Read the model definition and answer for the solid it produces. Units are mm, in the model's axes. Face numbers are marked on the shaded views. A direction names the side the tool comes from. Round coordinates to 2 decimals unless told otherwise and drop trailing zeros. Order: outer loops, then holes, each group sorted by start corner. A loop starts at its lowest first (then second) coordinate and runs counter-clockwise, first axis right, second up.
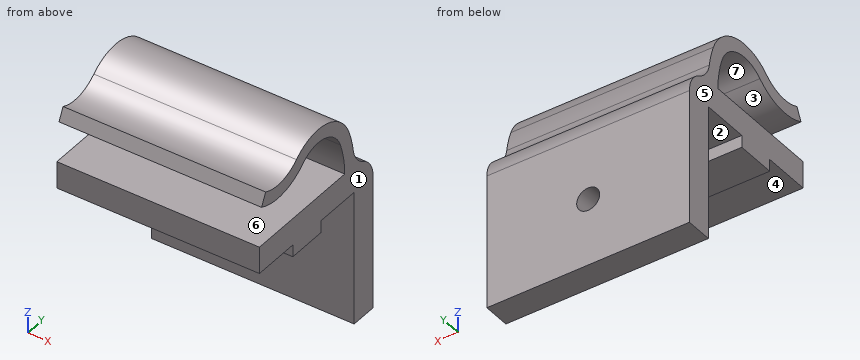
from build123d import *

# Parameters (mm, degrees)
PAD018_DEPTH    = 15
FILLET017_R     = 4
SKETCH077_R     = 1.7
POCKET041_DEPTH = 14.0010001


with BuildPart() as part:
    # Sketch076 → Pad018 (new body, symmetric)
    with BuildSketch(Plane.YZ):
        with BuildLine():
            Line((-2.95, 0), (2.95, 0))
            Line((2.95, 0), (2.95, 1.8))
            Line((2.95, 1.8), (10, 1.8))
            Line((10, -18.2), (10, 1.8))
            Line((14, -18.2), (10, -18.2))
            Line((14, 1.8), (14, -18.2))
            ThreePointArc((14, 1.8), (12.8284271247, 4.6284271247), (10, 5.8))
            ThreePointArc((10, 5.8), (9.7359108307, 8.6950147374), (8.9523612088, 11.4944617201))
            ThreePointArc((8.9523612088, 11.4944617201), (4.1074030924, 15.7943944981), (-2.1905894743, 14.2783698696))
            ThreePointArc((-8.6955362552, 13.3740094918), (-5.3083417089, 12.8571578981), (-2.1905894743, 14.2783698696))
            Line((-9.5491968047, 11.565345989), (-8.6955362552, 13.3740094918))
            ThreePointArc((-9.5491968047, 11.565345989), (-5.0329374097, 10.8762105308), (-0.8759344302, 12.7711598262))
            ThreePointArc((7.0833160577, 10.7826540051), (3.6226316889, 13.8540345608), (-0.8759344302, 12.7711598262))
            ThreePointArc((8, 5.8), (7.7689219768, 8.3331378952), (7.0833160577, 10.7826540051))
            Line((-10, 5.8), (8, 5.8))
            Line((-10, 5.8), (-10, 1.8))
            Line((-2.95, 1.8), (-10, 1.8))
            Line((-2.95, 0), (-2.95, 1.8))
        make_face()
    extrude(amount=PAD018_DEPTH, both=True)

    # Fillet017
    fillet017_edges = [part.edges().sort_by_distance(p)[0] for p in [
        (0, 10, 5.8),
    ]]
    fillet(fillet017_edges, radius=FILLET017_R)

    # Sketch077 → Pocket041 (cut, through all)
    with BuildSketch(Plane.XZ):
        with Locations((0, -8.2)):
            Circle(SKETCH077_R)
    extrude(amount=-POCKET041_DEPTH, mode=Mode.SUBTRACT)


solid = part.part
Q1. For a pull along Z with two mould halves and no side action, classify the marked faces 1, 2 and 3 as released by +Z, released by -Z, zero draft, split by the parting line, or undercut.
Outcome:
face 1: zero draft
face 2: released by -Z
face 3: undercut
Q2. For the marked faces 4, 5, 6 and 7, determine the directions among +Z, -Z, +X, -X, +Y, -Y from which every point of the face is accessible in a straight line to the end or side of a thin tool.
Outcome:
face 4: -Z, +X, -X, -Y
face 5: +Z, -Z, -X, +Y, -Y
face 6: +X, -X, -Y
face 7: +X, -X
Q3. A cutting plane is placed at A-A, the plane z = -8.2. Give the vertices of the cut face in (x, y), plus the area to 3 significant figures.
Outcome:
outline: (-15, 10) - (-1.7, 10) - (-1.7, 14) - (-15, 14) - close; (1.7, 10) - (15, 10) - (15, 14) - (1.7, 14) - close
area: 106 mm2
Q4. Flat-ended cylindrical pins translate along their axes: pin 1 (3 mm diameter, centred on x = -2, y = 4, fed in from -Z); pin 2 (4.5 mm diameter, centred on x = 0, z = -8.2, fed in from -Y); pin 3 (12 mm diameter, centred on y = -7, z = -1, fed in from -X); pin 4 (0.9 mm diameter, centred on x = 1.5, z = 1, fed in from -Y). Find the tip coordinate at first contact, or state that the pin passes through.
Outcome:
pin 1: stops at z = 0
pin 2: stops at y = 10
pin 3: stops at x = -15
pin 4: stops at y = -2.95
Q5. A cutting plane is placed at B-B, the plane y = 5.75. Give the vertices of the cut face in (x, z).
Outcome:
outline: (-15, 1.8) - (15, 1.8) - (15, 5.8) - (-15, 5.8) - close; (-15, 12.72) - (15, 12.72) - (15, 15.16) - (-15, 15.16) - close
Q6. A cutting plane is placed at D-D, the plane z = 3.5. Give the vertices of the cut face in (x, y), plus the area to 3 significant figures.
Outcome:
outline: (-15, -10) - (15, -10) - (15, 13.62) - (-15, 13.62) - close
area: 709 mm2
Q7. Straight lines are drawn through the part: probe 1 along Y at (x, z) = (-4, -6.5); probe 2 along Z at (x, y) = (11, 5); probe 3 along Y at (x, z) = (-3, 12). For each, find the intervals that lie inside material, in ascending order.
Outcome:
probe 1: y = 10 to 14
probe 2: z = 1.8 to 5.8, 13.28 to 15.51
probe 3: y = -9.34 to -1.92, 6.41 to 8.74
Q8. A cutting plane is placed at C-C, the plane z = -15. Give the vertices of the cut face in (x, y).
Outcome:
outline: (-15, 10) - (15, 10) - (15, 14) - (-15, 14) - close
